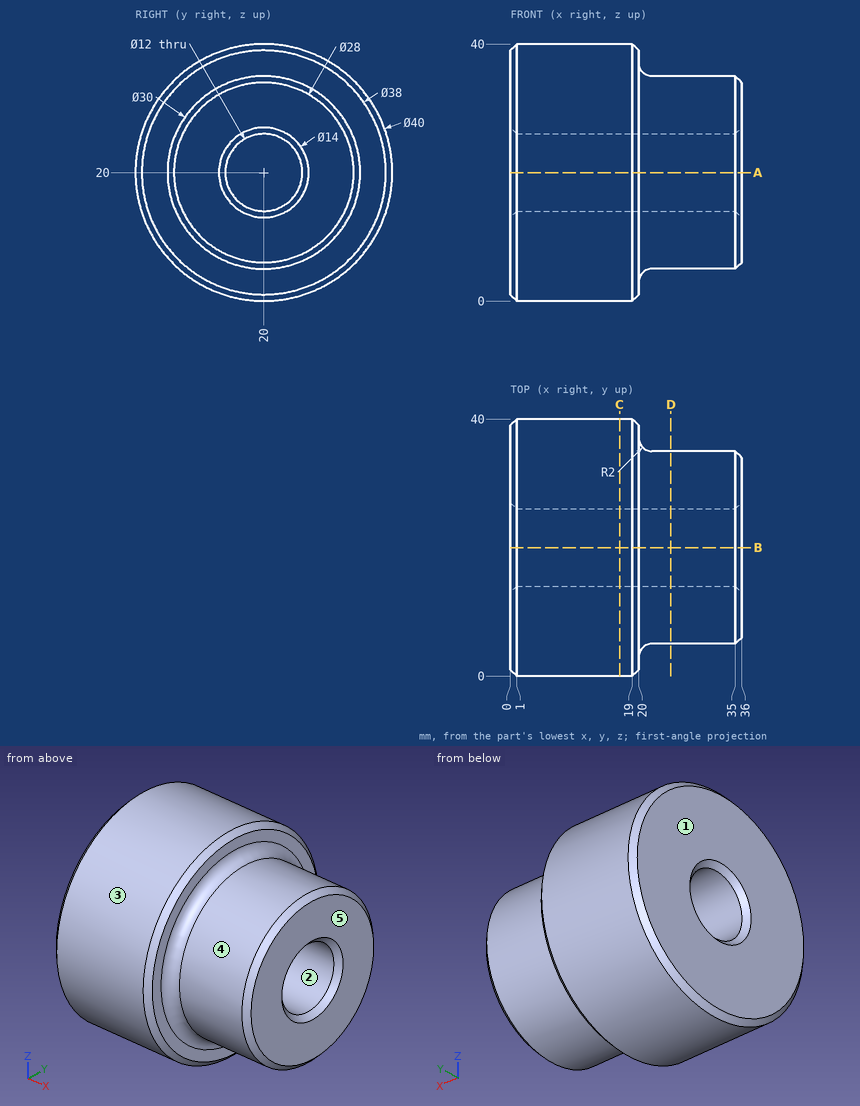
Drawing for the job (mm, zero at the part's lowest x, y, z). A direction names the side the tool comes from. Round coordinates to 2 decimals unless told otherwise and drop trailing zeros. Loops run counter-clockwise (first coordinate to the right, second up) from the corner with the lowest first, then second, coordinate; pieces in that order, holes last.
1. Wall check: probe 1 along Z at (x, y) = (9, 20); probe 2 along Y at (x, z) = (15, 19.5); probe 3 along Z at (x, y) = (3.5, 21). Give the ranges that are in metal, low to high.
Check values:
probe 1: z = 0 to 14, 26 to 40
probe 2: y = 0.01 to 14.02, 25.98 to 39.99
probe 3: z = 0.03 to 14.08, 25.92 to 39.97
2. Band-saw the part on A-A, the plane z = 20. List the corners of the cut face in (x, y).
Check values:
outline: (0, 1) - (1, 0) - (19, 0) - (20, 1) - (20, 3) arc R2 cw to (22, 5) - (35, 5) - (36, 6) - (36, 13) - (35, 14) - (1, 14) - (0, 13) - close; (0, 27) - (1, 26) - (35, 26) - (36, 27) - (36, 34) - (35, 35) - (22, 35) arc R2 cw to (20, 37) - (20, 39) - (19, 40) - (1, 40) - (0, 39) - close
3. Mould opens along Z. For the marked faces 1, 2 and 3 say: +Z half, -Z half, draft (parallel to the pull), parting line (faces both ways), or undercut.
Check values:
face 1: draft
face 2: undercut
face 3: parting line
4. Drop flat-ended pins along their axis: P1, Ø6, axis at x = 13.5, z = 9, coming from the -Y side; P2, Ø1.5, axis at x = 6, z = 9.5, coming from the +Y side; P3, Ø4, axis at y = 28, z = 6, coming from the +X side; P4, Ø11, axis at y = 20, z = 20, coming from the +X side. Give the stop position or say it passes through.
Check values:
P1: stops at y = 1.67
P2: stops at y = 37.46
P3: stops at x = 35.88
P4: passes through
5. Band-saw the part on D-D, the plane x = 25. List the corners of the cut face in (y, z), and give its area (3 significant figures).
Check values:
outline: circle Ø30 at (20, 20); hole circle Ø12 at (20, 20)
area: 594 mm2
6. Tool access for the marked faces 4 and 5: list every direction of +Z, -Z, +X, -X, +Y, -Y with a clear straight run to the whole face (end or side of a thin tool).
Check values:
face 4: +X
face 5: +Z, -Z, +X, +Y, -Y
7. Band-saw the part on C-C, the plane x = 17. List the corners of the cut face in (y, z).
Check values:
outline: circle Ø40 at (20, 20); hole circle Ø12 at (20, 20)
